from build123d import *

# Parameters (mm, degrees)
BOSS_EXTRUDE1_DEPTH           = 1.25
SKETCH2_R                     = 0.5
BOSS_EXTRUDE2_DEPTH           = 2
BOSS_EXTRUDE2_DRAFT           = 5
BOSS_EXTRUDE2_PROFILE_2_DEPTH = 2
BOSS_EXTRUDE2_PROFILE_2_DRAFT = 5
BOSS_EXTRUDE2_PROFILE_3_DEPTH = 2
BOSS_EXTRUDE2_PROFILE_3_DRAFT = 5
BOSS_EXTRUDE2_PROFILE_4_DEPTH = 2
BOSS_EXTRUDE2_PROFILE_4_DRAFT = 5
BOSS_EXTRUDE3_REACH           = 28.514
BOSS_EXTRUDE3_END_RADIUS      = 10.5
SKETCH5_RX                    = 3
SKETCH5_RY                    = 2
FILLET1_START                 = -1.25
FILLET1_DEPTH                 = 2.5


with BuildPart() as part:
    # Sketch1 → Boss-Extrude1 (new, symmetric)
    with BuildSketch(Plane.XY):
        with BuildLine():
            Line((-10.307764064, 2), (-20.307764064, 2))
            Line((-20.307764064, 2), (-20.307764064, -2))
            Line((-20.307764064, -2), (-10.307764064, -2))
            ThreePointArc((-10.307764064, -2), (-10.5, 0), (-10.307764064, 2))
        make_face()
        with BuildLine():
            Line((1.74e-07, 10.5), (1.74e-07, 6.5))
            ThreePointArc((1.74e-07, 6.5), (-6.5, 0), (1.74e-07, -6.5))
            Line((1.74e-07, -6.5), (1.74e-07, -10.5))
            ThreePointArc((1.74e-07, -10.5), (-10.5, 0), (1.74e-07, 10.5))
        make_face()
        with BuildLine():
            ThreePointArc((1.74e-07, 10.5), (-0.626113962, 10.481315819), (-1.249999826, 10.425329752))
            Line((-1.249999826, 10.425329752), (-1.249999826, 6.5))
            Line((-1.249999826, 6.5), (1.74e-07, 6.5))
            Line((1.74e-07, 6.5), (1.74e-07, 10.5))
        make_face()
        with BuildLine():
            Line((-1.249999826, -6.5), (-1.249999826, -10.425329752))
            ThreePointArc((-1.249999826, -10.425329752), (-0.626113962, -10.481315819), (1.74e-07, -10.5))
            Line((1.74e-07, -10.5), (1.74e-07, -6.5))
            Line((1.74e-07, -6.5), (-1.249999826, -6.5))
        make_face()
    extrude(amount=BOSS_EXTRUDE1_DEPTH, both=True)


with BuildPart() as boss_extrude2_tool:
    # Sketch2 → Boss-Extrude2 (with draft: the straight prism first)
    with BuildSketch(Plane(origin=(0, 2, 0), x_dir=(1, 0, 0), z_dir=(0, 1, 0))):
        with Locations((-19.307764064, 0)):
            Circle(SKETCH2_R)
    extrude(amount=BOSS_EXTRUDE2_DEPTH)
    # Boss-Extrude2: the draft: its side faces are tilted about the plane it starts from
    boss_extrude2_sides = [boss_extrude2_tool.faces().sort_by_distance(p)[0] for p in [
        (-19.807764064, 3, 0),
    ]]
    draft(boss_extrude2_sides, Plane(origin=(0, 2, 0), x_dir=(1, 0, 0), z_dir=(0, 1, 0)), BOSS_EXTRUDE2_DRAFT)


with BuildPart() as part_1:
    add(part.part)

    # Boss-Extrude2: add boss_extrude2_tool
    add(boss_extrude2_tool.part)


with BuildPart() as boss_extrude2_profile_2_tool:
    # Sketch2 → Boss-Extrude2 profile 2 (with draft: the straight prism first)
    with BuildSketch(Plane(origin=(0, 2, 0), x_dir=(1, 0, 0), z_dir=(0, 1, 0))):
        with Locations((-17.207764064, 0)):
            Circle(SKETCH2_R)
    extrude(amount=BOSS_EXTRUDE2_PROFILE_2_DEPTH)
    # Boss-Extrude2 profile 2: the draft: its side faces are tilted about the plane it starts from
    boss_extrude2_profile_2_sides = [boss_extrude2_profile_2_tool.faces().sort_by_distance(p)[0] for p in [
        (-17.707764064, 3, 0),
    ]]
    draft(boss_extrude2_profile_2_sides, Plane(origin=(0, 2, 0), x_dir=(1, 0, 0), z_dir=(0, 1, 0)), BOSS_EXTRUDE2_PROFILE_2_DRAFT)


with BuildPart() as part_2:
    add(part_1.part)

    # Boss-Extrude2 profile 2: add boss_extrude2_profile_2_tool
    add(boss_extrude2_profile_2_tool.part)


with BuildPart() as boss_extrude2_profile_3_tool:
    # Sketch2 → Boss-Extrude2 profile 3 (with draft: the straight prism first)
    with BuildSketch(Plane(origin=(0, 2, 0), x_dir=(1, 0, 0), z_dir=(0, 1, 0))):
        with Locations((-15.107764064, 0)):
            Circle(SKETCH2_R)
    extrude(amount=BOSS_EXTRUDE2_PROFILE_3_DEPTH)
    # Boss-Extrude2 profile 3: the draft: its side faces are tilted about the plane it starts from
    boss_extrude2_profile_3_sides = [boss_extrude2_profile_3_tool.faces().sort_by_distance(p)[0] for p in [
        (-15.607764064, 3, 0),
    ]]
    draft(boss_extrude2_profile_3_sides, Plane(origin=(0, 2, 0), x_dir=(1, 0, 0), z_dir=(0, 1, 0)), BOSS_EXTRUDE2_PROFILE_3_DRAFT)


with BuildPart() as part_3:
    add(part_2.part)

    # Boss-Extrude2 profile 3: add boss_extrude2_profile_3_tool
    add(boss_extrude2_profile_3_tool.part)


with BuildPart() as boss_extrude2_profile_4_tool:
    # Sketch2 → Boss-Extrude2 profile 4 (with draft: the straight prism first)
    with BuildSketch(Plane(origin=(0, 2, 0), x_dir=(1, 0, 0), z_dir=(0, 1, 0))):
        with Locations((-13.007764064, 0)):
            Circle(SKETCH2_R)
    extrude(amount=BOSS_EXTRUDE2_PROFILE_4_DEPTH)
    # Boss-Extrude2 profile 4: the draft: its side faces are tilted about the plane it starts from
    boss_extrude2_profile_4_sides = [boss_extrude2_profile_4_tool.faces().sort_by_distance(p)[0] for p in [
        (-13.507764064, 3, 0),
    ]]
    draft(boss_extrude2_profile_4_sides, Plane(origin=(0, 2, 0), x_dir=(1, 0, 0), z_dir=(0, 1, 0)), BOSS_EXTRUDE2_PROFILE_4_DRAFT)


with BuildPart() as part_4:
    add(part_3.part)

    # Boss-Extrude2 profile 4: add boss_extrude2_profile_4_tool
    add(boss_extrude2_profile_4_tool.part)

    # Boss-Extrude3: up to this cylinder (the profile starts inside it)
    boss_extrude3_end = Plane(origin=(0, 0, 0), z_dir=(0, 0, -1)) * Cylinder(BOSS_EXTRUDE3_END_RADIUS, 79.028, mode=Mode.PRIVATE)
    # Sketch5 → Boss-Extrude3 (add, up to the surface)
    with BuildSketch(Plane(origin=(0, 6.5, 0), x_dir=(1, 0, 0), z_dir=(0, 1, 0)), mode=Mode.PRIVATE) as boss_extrude3_sk1:
        with Locations((0, 0)):
            Ellipse(SKETCH5_RX, SKETCH5_RY)
    boss_extrude3_tool1 = extrude(boss_extrude3_sk1.sketch, amount=BOSS_EXTRUDE3_REACH, mode=Mode.PRIVATE) & boss_extrude3_end
    boss_extrude3 = boss_extrude3_tool1.solids().sort_by_distance((0, 6.5, 0))[0]
    add(boss_extrude3)

    # Mirror1: Boss-Extrude3 across plane
    add(boss_extrude3.mirror(Plane.ZX))

    # Fillet1: read off the stored shape, not the designer's step
    # Fillet1 outline → Fillet1 (add)
    with BuildSketch(Plane.XY.offset(FILLET1_START)):
        with BuildLine():
            add(Edge.make_bspline(
                [(-11.779218989, 2), (-10.654356635, 2), (-9.513984568, 4.442307692)],
                knots=[0, 0, 0, 1, 1, 1], degree=2, weights=[1, 0.843527392, 1]))
            Line((-11.779218989, 2), (-10.307764064, 2))
            ThreePointArc((-10.307764064, 2), (-9.985822271, 3.245512837), (-9.513984568, 4.442307692))
        make_face()
        with BuildLine():
            add(Edge.make_bspline(
                [(-9.513984568, -4.442307692), (-10.654356635, -2), (-11.779218989, -2)],
                knots=[0, 0, 0, 1, 1, 1], degree=2, weights=[1, 0.843527392, 1]))
            ThreePointArc((-9.513984568, -4.442307692), (-9.985822271, -3.245512837), (-10.307764064, -2))
            Line((-10.307764064, -2), (-11.779218989, -2))
        make_face()
    extrude(amount=FILLET1_DEPTH)


solid = part_4.part
The model under review builds one solid part; all positions refer to its coordinate system, in mm. A direction names the side the tool comes from. Coordinates: 2 decimals unless noted, no trailing zeros. Write each loop counter-clockwise with the first axis right and the second up, starting at its lowest first coordinate (ties: lowest second). Pieces come first, ordered by that corner, then holes. Notation, with made-up numbers: (-14.5, -4) - (-9.5, -4) arc R33 cw to (-9.5, 32) - close; hole circle Ø7 at (-32, -1.5). An arc over 180 degrees is marked (long way). Answer as a JSON object with one key per item and string values. Group by question number.
1. To check wall thickness, follow probe 1 along X at (y, z) = (0.25, -0.1); probe 2 along Z at (x, y) = (-5.75, -7.25); probe 3 along Y at (x, z) = (0.5, -1.15). State the ranges of each line that lie inside material, in increasing order.
2. Add section C-C (x = -8). Give the boundary of the cut face in (y, z), plus the area to 3 significant figures.
3. Add section B-B (y = 0). Give the boundary of the cut face in (x, z), plus the area to 3 significant figures.
4. Add section A-A (y = 2.5). Give the number of separate pieces and of enclosed holes in the cut face, plus the area to 3 significant figures.
5. Clearance check with flat-ended pins moving along their axes: pin 1 Ø2 at (x, y) = (-4, 2) entering from -Z; pin 2 Ø0.8 at (x, z) = (-15, 0.5) entering from +Y; pin 3 Ø3 at (x, y) = (-15, -0.5) entering from +Z; pin 4 Ø6 at (x, y) = (-6, 0) entering from -Z. State where each tip first meets the part, or that it passes through.
6. Mouldability with a two-part tool opening along Y and no side actions: class faces 4 (the face through (-6.5, 0.1, 0)), 5 (the face through (-20.308, 0, 0)), 6 (the face through (-18.926, 2.986, 0.158)), 7 (the face through (1, 6.5, 0)) as pulls with the +Y half, pulls with the -Y half, needs draft (parallel to the pull), parting line crosses it, or undercut.
7. Machinability: for faces 1 (the face through (-16, -2, 0)), 2 (the face through (1, -6.5, 0)), 3 (the face through (-16, 2, 0)), which of the approach directions +Z, -Z, +X, -X, +Y, -Y give a long, thin tool a straight path to every point of the face, cutting with its end or side? Answer none if there is none.
Findings:
{
 "1": {"probe 1": "-20.31 to -6.5", "probe 2": "-1.25 to 1.25", "probe 3": "-10.49 to -6.5, 6.5 to 10.49"},
 "2": {"outline": "(-6.8, -1.25) - (6.8, -1.25) - (6.8, 1.25) - (-6.8, 1.25) - close", "area": "34.0 mm²"},
 "3": {"outline": "(-20.31, -1.25) - (-6.5, -1.25) - (-6.5, 1.25) - (-20.31, 1.25) - close", "area": "34.5 mm²"},
 "4": {"separate pieces": "5", "enclosed holes": "0", "area": "14.6 mm²"},
 "5": {"pin 1": "through", "pin 2": "y = 4", "pin 3": "z = 1.25", "pin 4": "z = -1.25"},
 "6": {"face 4": "undercut", "face 5": "needs draft", "face 6": "pulls with the +Y half", "face 7": "undercut"},
 "7": {"face 1": "+Z, -Z, -X, -Y", "face 2": "+X", "face 3": "+Y"}
}
